```python
from build123d import *

# Parameters (mm, degrees)
F1_DEPTH = 25.4
F2_R     = 3.175
F3_R     = 6.35
F4_R     = 2.5
F5_DEPTH = 50.801
F6_R     = 1.5
F6_R_2   = 4
F7_DEPTH = 50.801
F9_DEPTH = 1


with BuildPart() as f1:
    # F0 (on Front) → F1 (new body, symmetric)
    with BuildSketch(Plane.XZ):
        Polygon((4.76258, 50.8), (0, 50.8), (0, 0), (50.8, 0), (50.8, 4.76258), (4.76258, 4.76258), align=None)
    extrude(amount=F1_DEPTH, both=True)

    # F2
    f2_edges = [f1.edges().sort_by_distance(p)[0] for p in [
        (4.76258, 0, 50.8),
        (50.8, 0, 4.76258),
    ]]
    fillet(f2_edges, radius=F2_R)

    # F3
    f3_edges = [f1.edges().sort_by_distance(p)[0] for p in [
        (4.76258, 0, 4.76258),
    ]]
    fillet(f3_edges, radius=F3_R)

    # F4 (on face) → F5 (cut, through all)
    with BuildSketch(Plane(origin=(0, 0, 0), x_dir=(1, 0, 0), z_dir=(0, 0, -1))):
        with Locations((10, 16)):
            Circle(F4_R)
        with Locations((42, 16)):
            Circle(F4_R)
        with Locations((42, -16)):
            Circle(F4_R)
        with Locations((10, -16)):
            Circle(F4_R)
    extrude(amount=-F5_DEPTH, mode=Mode.SUBTRACT)

    # F6 (on face) → F7 (cut, through all)
    with BuildSketch(Plane(origin=(0, 0, 0), x_dir=(0, -1, 0), z_dir=(-1, 0, 0))):
        with Locations((15.5, 45.15)):
            Circle(F6_R)
        with Locations((15.5, 14.15)):
            Circle(F6_R)
        with Locations((-15.5, 14.15)):
            Circle(F6_R)
        with Locations((-15.5, 45.15)):
            Circle(F6_R)
        with Locations((0, 29.65)):
            Circle(F6_R_2)
    extrude(amount=-F7_DEPTH, mode=Mode.SUBTRACT)

    # F8 (on face) → F9 (cut)
    with BuildSketch(Plane(origin=(0, 0, 0), x_dir=(1, 0, 0), z_dir=(0, 0, -1))):
        with BuildLine():
            Line((13.263, -25.4), (13.263, 25.4))
            Line((13.263, 25.4), (11.263, 25.4))
            Line((11.263, 25.4), (11.263, 18.157506))
            ThreePointArc((11.263, 18.157506), (12.168813, 17.243483), (12.5, 16))
            ThreePointArc((12.5, 16), (12.168813, 14.756517), (11.263, 13.842494))
            Line((11.263, 13.842494), (11.263, -13.842494))
            ThreePointArc((11.263, -13.842494), (12.168813, -14.756517), (12.5, -16))
            ThreePointArc((12.5, -16), (12.168813, -17.243483), (11.263, -18.157506))
            Line((11.263, -18.157506), (11.263, -25.4))
            Line((11.263, -25.4), (13.263, -25.4))
        make_face()
    extrude(amount=-F9_DEPTH, mode=Mode.SUBTRACT)


solid = f1.part
```
Model file for the job. Use its own axes, mm. A direction names the side the tool comes from. Coordinates: 2 decimals unless noted, no trailing zeros. Loops run counter-clockwise (first coordinate to the right, second up) from the corner with the lowest first, then second, coordinate; pieces in that order, holes last. Notation, with made-up numbers: (67, 53) - (77, 53) arc R21 cw to (77, 59) - close; hole circle Ø7 at (55.5, 49). An arc over 180 degrees is marked (long way). Answer as a JSON object with one key per item and string values. Group by question number.
(1) Cut at D-D (y = -16). Give the cut face in (x, z) (3 decimals).
(2) Tool access for faces 1 (the face through (44.31, 16.96, 2.35)), 2 (the face through (30, 0, 4.763)): list every direction of +Z, -Z, +X, -X, +Y, -Y with a clear straight run to the whole face (end or side of a thin tool).
(3) Flat gauge pins, fed straight in: pin 1 (10.5 mm diameter, centred on y = 0, z = 29.65, fed in from +X); pin 2 (6 mm diameter, centred on x = 10, y = 16, fed in from +Z); pin 3 (4 mm diameter, centred on x = 32.5, y = -6.5, fed in from +Z); pin 4 (2.5 mm diameter, centred on y = 15.5, z = 45.15, fed in from -X). Where does each tip first touch, or does it go through?
(4) Cut at A-A (y = 0). Give the cut face in (x, z) (3 decimals), then the cut area to 3 significant figures.
(5) Probe line 1 along Y through (x, z) = (10, 1.75); line 2 along Y through (x, z) = (1, 45); line 3 along X through (y, z) = (-22, 43). List the from-to ranges inside material, lowest first.
(6) Cut at C-C (z = 29.65). Give the cut face in (x, y), then the cut area to 3 significant figures.
(7) Two-plate mould, pull along X, no slides. Class faces 3 (the face through (4.763, 0, 25)), 4 (the face through (6, 0, 0)), 5 (the face through (12, 0, 1)), 6 (the face through (0, -6, 26)): released by +X, released by -X, zero draft, split by the parting line, or undercut.
(8) Cut at B-B (z = 45.15). Give the cut face in (x, y), then the cut area to 3 significant figures.
Geometry says:
{
 "1": {"outline": "(0, 0) - (7.5, 0) - (7.5, 5.89) arc R6.35 cw to (4.763, 11.113) - (4.763, 12.736) - (0, 12.736) - close; (0, 15.564) - (4.763, 15.564) - (4.763, 43.736) - (0, 43.736) - close; (0, 46.564) - (4.763, 46.564) - (4.763, 47.625) arc R3.175 ccw to (1.588, 50.8) - (0, 50.8) - close; (12.5, 1) - (13.263, 1) - (13.263, 0) - (39.5, 0) - (39.5, 4.763) - (12.5, 4.763) - close; (44.5, 0) - (50.8, 0) - (50.8, 1.588) arc R3.175 ccw to (47.625, 4.763) - (44.5, 4.763) - close"},
 "2": {"face 1": "+Z, -Z", "face 2": "+Z, +X, +Y, -Y"},
 "3": {"pin 1": "stops at x = 4.76", "pin 2": "stops at z = 6.27", "pin 3": "stops at z = 4.76", "pin 4": "passes through"},
 "4": {"outline": "(0, 0) - (11.263, 0) - (11.263, 1) - (13.263, 1) - (13.263, 0) - (50.8, 0) - (50.8, 1.588) arc R3.175 ccw to (47.625, 4.763) - (11.113, 4.763) arc R6.35 cw to (4.763, 11.113) - (4.763, 25.65) - (0, 25.65) - close; (0, 33.65) - (4.763, 33.65) - (4.763, 47.625) arc R3.175 ccw to (1.588, 50.8) - (0, 50.8) - close", "area": "425 mm^2"},
 "5": {"line 1": "y = -25.4 to -18.5, -13.5 to 13.5, 18.5 to 25.4", "line 2": "y = -25.4 to -16.99, -14.01 to 14.01, 16.99 to 25.4", "line 3": "x = 0 to 4.76"},
 "6": {"outline": "(0, -25.4) - (4.76, -25.4) - (4.76, -4) - (0, -4) - close; (0, 4) - (4.76, 4) - (4.76, 25.4) - (0, 25.4) - close", "area": "204 mm^2"},
 "7": {"face 3": "released by +X", "face 4": "zero draft", "face 5": "undercut", "face 6": "released by -X"},
 "8": {"outline": "(0, -25.4) - (4.76, -25.4) - (4.76, -17) - (0, -17) - close; (0, -14) - (4.76, -14) - (4.76, 14) - (0, 14) - close; (0, 17) - (4.76, 17) - (4.76, 25.4) - (0, 25.4) - close", "area": "213 mm^2"}
}
